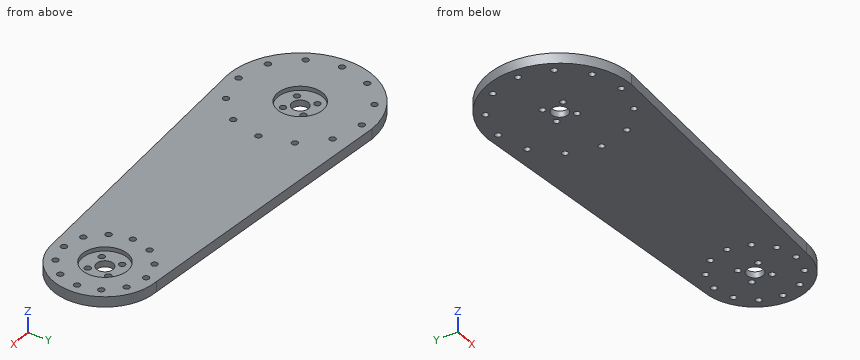
from build123d import *

# Parameters (mm, degrees)
EXTRUDE_3_DEPTH     = 5
SKETCH_4_R          = 4
SKETCH_4_R_2        = 1.5
CUT_EXTRUDE_3_DEPTH = 5
SKETCH_5_R          = 11
CUT_EXTRUDE_4_DEPTH = 2
SKETCH_6_R          = 1.5
CUT_EXTRUDE_6_DEPTH = 169.745370307


with BuildPart() as part:
    # 草图1 → 凸台-拉伸3 (new body)
    with BuildSketch(Plane.XY):
        with BuildLine():
            Line((140, 25), (0, 35))
            ThreePointArc((0, 35), (-35, 0), (0, -35))
            Line((0, -35), (140, -25))
            ThreePointArc((140, -25), (165, 0), (140, 25))
        make_face()
    extrude(amount=EXTRUDE_3_DEPTH)

    # 草图4 → 切除-拉伸3 (cut)
    with BuildSketch(Plane.XY.offset(5)):
        with Locations((140, 0)):
            Circle(SKETCH_4_R)
        Circle(SKETCH_4_R)
        with BuildLine():
            Line((-5, -3.5), (-5, -5))
            Line((-5, -5), (-3.5, -5))
            ThreePointArc((-3.5, -5), (-3.939339828, -3.939339828), (-5, -3.5))
        make_face()
        with BuildLine():
            Line((-3.5, -5), (-5, -5))
            Line((-5, -5), (-5, -3.5))
            ThreePointArc((-5, -3.5), (-6.060660172, -6.060660172), (-3.5, -5))
        make_face()
        with Locations((135, 5)):
            Circle(SKETCH_4_R_2)
        with Locations((135, -5)):
            Circle(SKETCH_4_R_2)
        with Locations((145, -5)):
            Circle(SKETCH_4_R_2)
        with Locations((145, 5)):
            Circle(SKETCH_4_R_2)
        with Locations((-5, 5)):
            Circle(SKETCH_4_R_2)
        with Locations((5, 5)):
            Circle(SKETCH_4_R_2)
        with Locations((5, -5)):
            Circle(SKETCH_4_R_2)
    extrude(amount=-CUT_EXTRUDE_3_DEPTH, mode=Mode.SUBTRACT)

    # 草图5 → 切除-拉伸4 (cut)
    with BuildSketch(Plane.XY.offset(5)):
        Circle(SKETCH_5_R)
        with Locations((140, 0)):
            Circle(SKETCH_5_R)
    extrude(amount=-CUT_EXTRUDE_4_DEPTH, mode=Mode.SUBTRACT)

    # 草图6 → 切除-拉伸6 (cut, through all)
    with BuildSketch(Plane.XY.offset(5)):
        with Locations((0, 30)):
            Circle(SKETCH_6_R)
        with Locations((15, 25.980762114)):
            Circle(SKETCH_6_R)
        with Locations((25.980762114, 15)):
            Circle(SKETCH_6_R)
        with Locations((30, 0)):
            Circle(SKETCH_6_R)
        with Locations((25.980762114, -15)):
            Circle(SKETCH_6_R)
        with Locations((15, -25.980762114)):
            Circle(SKETCH_6_R)
        with Locations((0, -30)):
            Circle(SKETCH_6_R)
        with Locations((-15, -25.980762114)):
            Circle(SKETCH_6_R)
        with Locations((-25.980762114, -15)):
            Circle(SKETCH_6_R)
        with Locations((-30, 0)):
            Circle(SKETCH_6_R)
        with Locations((-25.980762114, 15)):
            Circle(SKETCH_6_R)
        with Locations((-15, 25.980762114)):
            Circle(SKETCH_6_R)
        with Locations((140, 20)):
            Circle(SKETCH_6_R)
        with Locations((150, 17.320508076)):
            Circle(SKETCH_6_R)
        with Locations((157.320508076, 10)):
            Circle(SKETCH_6_R)
        with Locations((160, 0)):
            Circle(SKETCH_6_R)
        with Locations((157.320508076, -10)):
            Circle(SKETCH_6_R)
        with Locations((150, -17.320508076)):
            Circle(SKETCH_6_R)
        with Locations((140, -20)):
            Circle(SKETCH_6_R)
        with Locations((130, -17.320508076)):
            Circle(SKETCH_6_R)
        with Locations((122.679491924, -10)):
            Circle(SKETCH_6_R)
        with Locations((120, 0)):
            Circle(SKETCH_6_R)
        with Locations((122.679491924, 10)):
            Circle(SKETCH_6_R)
        with Locations((130, 17.320508076)):
            Circle(SKETCH_6_R)
    extrude(amount=-CUT_EXTRUDE_6_DEPTH, mode=Mode.SUBTRACT)


solid = part.part
Here's how the part is built. I have some questions about the finished solid (model axes, mm). Round coordinates to 2 decimals unless told otherwise and drop trailing zeros. Order: outer loops, then holes, each group sorted by start corner. A loop starts at its lowest first (then second) coordinate and runs counter-clockwise, first axis right, second up. Notation, with made-up numbers: M 10,57 L 41,57 A20 cw 41,70 Z; hole C 29.25,42 d6. An arc over 180 degrees is marked long. Return JSON: item names as keys, results as strings. Group by question number.
1. Please list where these lines run through material, in increasing order: probe 1 along Y at (x, z) = (134, 2.55); probe 2 along Y at (x, z) = (135, 1.8); probe 3 along X at (y, z) = (-9.5, 1.6).
2. If we section it at C-C on x = 85.5: List the corners of the cut face in (y, z) for me, then the cut area to 3 significant figures.
3. I'm going to push flat-ended pins straight in: pin 1 Ø1.8 at (x, y) = (-25.98, 15) entering from +Z; pin 2 Ø1 at (x, z) = (11.5, 4.5) entering from -Y; pin 3 Ø1.5 at (y, z) = (10, 3) entering from +X; pin 4 Ø2 at (y, z) = (-3.5, 3) entering from -X. Where does each tip first touch, or does it pass through?
4. If we section it at B-B on x = 40: List the corners of the cut face in (y, z) for me, then the cut area to 3 significant figures.
5. If we section it at A-A on x = -9: List the corners of the cut face in (y, z) for me.
Reply:
{
 "1": {"probe 1": "-25.43 to -6.12, -3.88 to 3.88, 6.12 to 25.43", "probe 2": "-25.36 to -6.5, -3.5 to 3.5, 6.5 to 25.36", "probe 3": "-33.69 to 121.27, 124.09 to 155.91, 158.73 to 163.12"},
 "2": {"outline": "M -28.89,0 L 28.89,0 L 28.89,5 L -28.89,5 Z", "area": "289 mm^2"},
 "3": {"pin 1": "through", "pin 2": "y = -34.21", "pin 3": "x = 163.23", "pin 4": "x = -34.91"},
 "4": {"outline": "M -32.14,0 L 32.14,0 L 32.14,5 L -32.14,5 Z", "area": "321 mm^2"},
 "5": {"outline": "M -33.82,0 L 33.82,0 L 33.82,5 L 6.32,5 L 6.32,3 L -6.32,3 L -6.32,5 L -33.82,5 Z"}
}
